The listing builds one solid part. Answer for the finished solid, in the listing's coordinates (mm). A direction names the side the tool comes from. Give positions to 0.01 mm unless a question says otherwise; leave off trailing zeros. Order: outer loops, then holes, each group sorted by start corner. A loop starts at its lowest first (then second) coordinate and runs counter-clockwise, first axis right, second up. Notation, with made-up numbers: (-24, 7) - (34, 7) arc R30 ccw to (34, 36) - close; hole circle Ø8 at (39.25, -24.75). An arc over 180 degrees is marked (long way). Write each question's results on one line, items separated by ' | '. Start each with the question number.
1. Section A-A (z = 21) is taken. Give the vertices of the cut face in (x, y).
2. Section C-C (x = -50) is taken. Give the vertices of the cut face in (y, z).
3. Which of the six approach directions +Z, -Z, +X, -X, +Y, -Y give full straight-line access (tool end or side, diameter ignored) to faces 1 (the face through (48, -4, 8)), 2 (the face through (-36.514, -3.944, 26.32)), 3 (the face through (25.789, -4.056, 9.804))?
4. Determine the mould class of faces 4 (the face through (66, -4, 10)), 5 (the face through (-32, -4, 15)), 6 (the face through (27.5, -4, 18)) for opening direction Y: released by +Y, released by -Y, zero draft, split by the parting line, or undercut.
5. Find the intervals of material crossed by L1, parallel to Y at x = -31.5, z = 19.5; L2, parallel to X at y = -6, z = 6.5; L3, parallel to X at y = -6, z = 9.5, in increasing order.
6. Section B-B (x = 65.25) is taken. Give the vertices of the cut face in (y, z), and give its area (3 significant figures).
7. Flat-ended cylindrical pins translate along their axes: pin 1 (4 mm diameter, centred on y = -4, z = 16.5, fed in from -X); pin 2 (2 mm diameter, centred on x = -31.5, y = -4, fed in from -Z); pin 3 (2.5 mm diameter, centred on y = -2.5, z = 19.5, fed in from +X). Find the tip coordinate at first contact, or state that the pin passes through.
from build123d import *

# Parameters (mm, degrees)
F0_R     = 1.75
F1_DEPTH = 8
F2_R     = 6
F3_R     = 3.5
F4_DEPTH = 4
F5_R     = 1.4
F6_DEPTH = 15
F7_R     = 1.4
F8_DEPTH = 15


# Not quite as in the source:
# - a feature names something its author has since deleted; it is built from what else it names


with BuildPart() as f1:
    # F0 (on Front) → F1 (new body)
    with BuildSketch(Plane.XZ):
        with BuildLine():
            Line((-75.25, 0), (0, 0))
            Line((0, 0), (75.25, 0))
            Line((75.25, 0), (75.25, -8))
            ThreePointArc((75.25, -8), (79.25, -12), (83.25, -8))
            Line((83.25, -8), (83.25, 8))
            Line((83.25, 8), (71.25, 8))
            ThreePointArc((71.25, 8), (65.25, 14), (59.25, 8))
            Line((59.25, 8), (35.5, 8))
            Line((35.5, 8), (35.5, 22.5358983849))
            Line((35.5, 22.5358983849), (35.5, 30))
            Line((35.5, 30), (27.5, 30))
            Line((27.5, 30), (27.5, 22.5358983849))
            Line((27.5, 22.5358983849), (27.5, 8))
            Line((27.5, 8), (0, 8))
            Line((0, 8), (-27.5, 8))
            Line((-27.5, 8), (-27.5, 22.5358983849))
            Line((-27.5, 22.5358983849), (-27.5, 30))
            Line((-27.5, 30), (-35.5, 30))
            Line((-35.5, 30), (-35.5, 22.5358983849))
            Line((-35.5, 22.5358983849), (-35.5, 13.9529404499))
            ThreePointArc((-35.5, 13.9529404499), (-40.2186269666, 12.5), (-42.25, 8))
            Line((-42.25, 8), (-83.25, 8))
            Line((-83.25, 8), (-83.25, -8))
            ThreePointArc((-83.25, -8), (-79.25, -12), (-75.25, -8))
            Line((-75.25, -8), (-75.25, 0))
        make_face()
        with Locations((-36.25, 8)):
            Circle(F0_R, mode=Mode.SUBTRACT)
        with Locations((65.25, 8)):
            Circle(F0_R, mode=Mode.SUBTRACT)
        Polygon((-37.5, 30), (-35.5, 22.5358983849), (-35.5, 30), align=None)
        Polygon((-25.5, 30), (-27.5, 30), (-27.5, 22.5358983849), align=None)
        Polygon((27.5, 22.5358983849), (27.5, 30), (25.5, 30), align=None)
        Polygon((35.5, 30), (35.5, 22.5358983849), (37.5, 30), align=None)
    extrude(amount=F1_DEPTH)

    # F2
    f2_edges = [f1.edges().sort_by_distance(p)[0] for p in [
        (59.25, -4, 8),
        (71.25, -4, 8),
        (83.25, -4, 8),
        (-83.25, -4, 8),
        (-35.5, -4, 13.95294),
        (-27.5, -4, 8),
        (27.5, -4, 8),
        (35.5, -4, 8),
        (-42.25, -4, 8),
    ]]
    fillet(f2_edges, radius=F2_R)

    # F3 (on face) → F4 (cut)
    with BuildSketch(Plane.XZ.offset(8)):
        with Locations((-36.25, 8)):
            Circle(F3_R)
        with Locations((65.25, 8)):
            Circle(F3_R)
    extrude(amount=-F4_DEPTH, mode=Mode.SUBTRACT)

    # F5 (on face) → F6 (cut)
    with BuildSketch(Plane.XY.offset(30)):
        with Locations((-31.5, -4)):
            Circle(F5_R)
    extrude(amount=-F6_DEPTH, mode=Mode.SUBTRACT)

    # F7 (on face) → F8 (cut)
    with BuildSketch(Plane.XY.offset(30)):
        with Locations((31.5, -4)):
            Circle(F7_R)
    extrude(amount=-F8_DEPTH, mode=Mode.SUBTRACT)


solid = f1.part
Reported:
1) outline: (-35.5, -8) - (-27.5, -8) - (-27.5, 0) - (-35.5, 0) - close; (27.5, -8) - (35.5, -8) - (35.5, 0) - (27.5, 0) - close; hole circle Ø2.8 at (-31.5, -4); hole circle Ø2.8 at (31.5, -4)
2) outline: (-8, 0) - (0, 0) - (0, 8) - (-8, 8) - close
3) face 1: +Z, +Y, -Y | face 2: -X, +Y, -Y | face 3: +Y, -Y
4) face 4: released by -Y | face 5: undercut | face 6: zero draft
5) L1: -8 to -5.4, -2.6 to 0 | L2: -81.22 to -39.41, -33.09 to 62.09, 68.41 to 81.22 | L3: -42.67 to -39.41, -33.09 to -25.47, 25.47 to 37.53, 58.83 to 62.09, 68.41 to 71.67
6) outline: (-8, 0) - (0, 0) - (0, 6.25) - (-4, 6.25) - (-4, 4.5) - (-8, 4.5) - close; (-8, 11.5) - (-4, 11.5) - (-4, 9.75) - (0, 9.75) - (0, 14) - (-8, 14) - close | area: 70.0 mm²
7) pin 1: x = -37.31 | pin 2: z = 0 | pin 3: x = 35.5
